```python
from build123d import *

# Parameters (mm, degrees)
F0_R     = 3.2677789254
F0_R_2   = 3.5
F1_DEPTH = 3


# Not quite as in the source:
# - a feature names something its author has since deleted; it is built from what else it names


with BuildPart() as f1:
    # F0 (on Top) → F1 (new body)
    with BuildSketch(Plane.XY):
        with BuildLine():
            ThreePointArc((-12.185161002, 20.1667081565), (-10.2249151213, 27.7991061308), (-12.9275786797, 35.2012458513))
            ThreePointArc((-12.9275786797, 35.2012458513), (-16.80912748, 33.5216830329), (-20.4768659437, 31.4157279261))
            ThreePointArc((-20.4768659437, 31.4157279261), (-16.1164151017, 18.0121200855), (-22.876226066, 5.6438061173))
            ThreePointArc((-22.876226066, 5.6438061173), (-26.8870432753, 12.4268296367), (-34.0322181964, 15.7498610989))
            ThreePointArc((-34.0322181964, 15.7498610989), (-35.5892574163, 11.8175613624), (-36.6936050187, 7.7349434862))
            ThreePointArc((-36.6936050187, 7.7349434862), (-24.1325186628, 1.3404658492), (-20.1667081565, -12.185161002))
            ThreePointArc((-20.1667081565, -12.185161002), (-27.7991061308, -10.2249151213), (-35.2012458513, -12.9275786797))
            ThreePointArc((-35.2012458513, -12.9275786797), (-33.5216830329, -16.80912748), (-31.4157279261, -20.4768659437))
            ThreePointArc((-31.4157279261, -20.4768659437), (-18.0121200855, -16.1164151017), (-5.6438061173, -22.876226066))
            ThreePointArc((-5.6438061173, -22.876226066), (-12.4268296367, -26.8870432753), (-15.7498610989, -34.0322181964))
            ThreePointArc((-15.7498610989, -34.0322181964), (-11.8175613624, -35.5892574163), (-7.7349434862, -36.6936050187))
            ThreePointArc((-7.7349434862, -36.6936050187), (-1.3404658492, -24.1325186628), (12.185161002, -20.1667081565))
            ThreePointArc((12.185161002, -20.1667081565), (10.2249151213, -27.7991061308), (12.9275786797, -35.2012458513))
            ThreePointArc((12.9275786797, -35.2012458513), (16.80912748, -33.5216830329), (20.4768659437, -31.4157279261))
            ThreePointArc((20.4768659437, -31.4157279261), (16.1164151017, -18.0121200855), (22.876226066, -5.6438061173))
            ThreePointArc((22.876226066, -5.6438061173), (26.8870432753, -12.4268296367), (34.0322181964, -15.7498610989))
            ThreePointArc((34.0322181964, -15.7498610989), (35.5892574163, -11.8175613624), (36.6936050187, -7.7349434862))
            ThreePointArc((36.6936050187, -7.7349434862), (24.1325186628, -1.3404658492), (20.1667081565, 12.185161002))
            ThreePointArc((20.1667081565, 12.185161002), (21.2681317348, 11.5765458519), (22.4221424931, 11.0747436302))
            ThreePointArc((22.4221424931, 11.0747436302), (29.051621985, 10.3463660778), (35.2012458513, 12.9275786797))
            ThreePointArc((35.2012458513, 12.9275786797), (33.5216830329, 16.80912748), (31.4157279261, 20.4768659437))
            ThreePointArc((31.4157279261, 20.4768659437), (18.0121200855, 16.1164151017), (5.6438061173, 22.876226066))
            ThreePointArc((5.6438061173, 22.876226066), (12.4268296367, 26.8870432753), (15.7498610989, 34.0322181964))
            ThreePointArc((15.7498610989, 34.0322181964), (11.8175613624, 35.5892574163), (7.7349434862, 36.6936050187))
            ThreePointArc((7.7349434862, 36.6936050187), (1.3404658492, 24.1325186628), (-12.185161002, 20.1667081565))
        make_face()
        with Locations((-6.3489950769, -8.7386420371)):
            Circle(F0_R, mode=Mode.SUBTRACT)
        with Locations((6.3489950769, -8.7386420371)):
            Circle(F0_R, mode=Mode.SUBTRACT)
        with Locations((-10.2728898289, 3.3378642426)):
            Circle(F0_R, mode=Mode.SUBTRACT)
        Circle(F0_R_2, mode=Mode.SUBTRACT)
        with Locations((10.2728898289, 3.3378642426)):
            Circle(F0_R, mode=Mode.SUBTRACT)
        with Locations((0, 10.8015555888)):
            Circle(F0_R, mode=Mode.SUBTRACT)
    extrude(amount=F1_DEPTH)


solid = f1.part
```
The listing builds one solid part. Answer for the finished solid, in the listing's coordinates (mm). Round coordinates to 2 decimals unless told otherwise and drop trailing zeros. Loops run counter-clockwise (first coordinate to the right, second up) from the corner with the lowest first, then second, coordinate; pieces in that order, holes last. Notation, with made-up numbers: (83, 87) - (98, 87) arc R17 cw to (98, 95) - close; hole circle Ø11 at (80, -14). An arc over 180 degrees is marked (long way). Use one line per item in the form item = value. Start each with the question number.
1. The part is cut by section A-A on x = 26. Determine the outline of the cut face in (y, z).
2. For a pull along Y with two mould halves and no side action, classify faces 1 (the face through (-11.87, -35.57, 1.48)), 2 (the face through (-16.756, 33.548, 1.479)), 3 (the face through (10.22, -27.69, 1.48)) as pulls with the +Y half, pulls with the -Y half, needs draft (parallel to the pull), parting line crosses it, or undercut.
3. The part is cut by section D-D on y = 28.5. Determine the outline of the cut face in (x, z).
4. Given pin 1 Ø1 at (x, z) = (18, 2) entering from -Y, flat-ended and moving along its own axis, determine where the tip first touches the part or whether it passes through.
5. The part is cut by section B-B on y = 1.5. Determine the outline of the cut face in (x, z), then the cut area to 3 significant figures.
6. Consider line 1 (Y direction, x = 12.5, z = 0.85); line 2 (X direction, y = 2, z = 2.65); line 3 (Y direction, x = 0, z = 1.75). Determine where each line is inside the solid, lowest interval first. Write a range as [from, to].
7. The part is cut by section C-C on z = 1.95. Give the number of separate pieces and of enclosed holes in the cut face, then the cut area to 3 significant figures.
Geometry check:
q1.outline = (-11.54, 0) - (-3.27, 0) - (-3.27, 3) - (-11.54, 3) - close; (10.26, 0) - (17.21, 0) - (17.21, 3) - (10.26, 3) - close
q2.face_1 = pulls with the -Y half
q2.face_2 = pulls with the +Y half
q2.face_3 = undercut
q3.outline = (-18.39, 0) - (-10.28, 0) - (-10.28, 3) - (-18.39, 3) - close; (5.13, 0) - (13.68, 0) - (13.68, 3) - (5.13, 3) - close
q4.pin_1 = -33.17
q5.outline = (-24.27, 0) - (-12.97, 0) - (-12.97, 3) - (-24.27, 3) - close; (-7.57, 0) - (-3.16, 0) - (-3.16, 3) - (-7.57, 3) - close; (3.16, 0) - (7.57, 0) - (7.57, 3) - (3.16, 3) - close; (12.97, 0) - (22.21, 0) - (22.21, 3) - (12.97, 3) - close
q5.area = 88.0 mm^2
q6.line_1 = [-34.61, 0.95], [5.73, 17.54], [26.97, 35.36]
q6.line_2 = [-24.71, -13.25], [-7.29, -2.87], [2.87, 7.29], [13.25, 21.94]
q6.line_3 = [-23.12, -3.5], [3.5, 7.53], [14.07, 23.12]
q7.separate_pieces = 1
q7.enclosed_holes = 6
q7.area = 2,190 mm^2
